Source: CAD feature listing. Evaluate the final solid. Frame: model axes, mm. Face numbers are marked on the shaded views. A direction names the side the tool comes from. Coordinates: 2 decimals unless noted, no trailing zeros. Loops run counter-clockwise (first coordinate to the right, second up) from the corner with the lowest first, then second, coordinate; pieces in that order, holes last. Notation, with made-up numbers: (56.5, 30.25) -> (92.5, 30.25) arc R19 ccw to (92.5, 41.25) -> close; hole circle Ø2 at (-39, 14.25). An arc over 180 degrees is marked (long way). Answer as a JSON object with one key per item and string values. Group by question number.
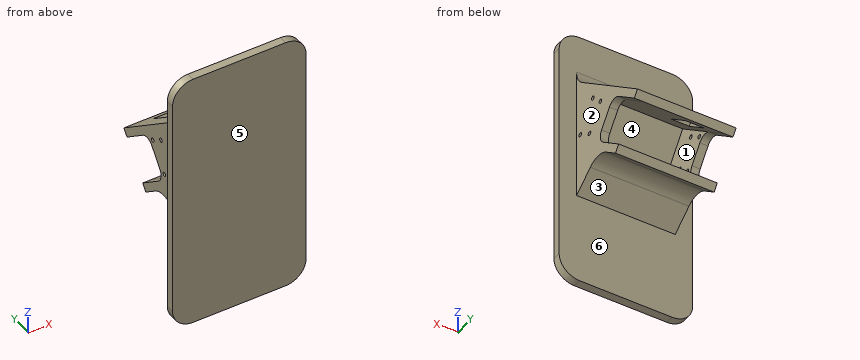
from build123d import *

# Parameters (mm, degrees)
BASE_PLATE_EXTRUDE_DEPTH    = 4
MOTORCASEEXTRUDE_DEPTH      = 24
MOTORCASEEXTRUDE_DEPTH_BACK = 24
SKETCH7_W                   = 40
SKETCH7_H                   = 20
CUT_EXTRUDE1_DEPTH          = 44
SKETCH9_W                   = 48
SKETCH9_H                   = 4
CUT_EXTRUDE2_DEPTH          = 28
FILLET_2_DEPTH              = 48
SKETCH11_W                  = 9
SKETCH11_H                  = 14
HOLE_FOR_WIRE_DEPTH         = 4
CUT_EXTRUDE3_REACH          = 14.5
SKETCH13_R                  = 1
CUT_EXTRUDE4_REACH          = 14.5
SKETCH14_R                  = 1


with BuildPart() as part:
    # Sketch1 → base_plate_extrude (new body)
    with BuildSketch(Plane(origin=(0, 0, 0), x_dir=(1, 0, 0), z_dir=(0, 1, 0))):
        with BuildLine():
            Line((-22.5, -63.5), (22.5, -63.5))
            ThreePointArc((22.5, -63.5), (29.571067812, -60.571067812), (32.5, -53.5))
            Line((32.5, -53.5), (32.5, 53.5))
            ThreePointArc((32.5, 53.5), (29.571067812, 60.571067812), (22.5, 63.5))
            Line((22.5, 63.5), (-22.5, 63.5))
            ThreePointArc((-22.5, 63.5), (-29.571067812, 60.571067812), (-32.5, 53.5))
            Line((-32.5, 53.5), (-32.5, -53.5))
            ThreePointArc((-32.5, -53.5), (-29.571067812, -60.571067812), (-22.5, -63.5))
        make_face()
    extrude(amount=BASE_PLATE_EXTRUDE_DEPTH)

    # Sketch5 → MotorCaseExtrude (add, two sides)
    with BuildSketch(Plane.ZY) as motorcaseextrude_sk:
        with BuildLine():
            Line((31.511856475, 15.127443917), (2.840895128, 53.623884992))
            Line((2.840895128, 53.623884992), (-19.615362165, 36.89915754))
            Line((-19.615362165, 36.89915754), (-11.812816694, 26.422695717))
            ThreePointArc((-11.812816694, 26.422695717), (-9.832908585, 20.44957877), (-11.812816694, 14.476461823))
            Line((-11.812816694, 14.476461823), (-19.615362165, 4))
            Line((-19.615362165, 4), (39.799233322, 4))
            Line((39.799233322, 4), (44.820226981, 4))
            ThreePointArc((44.820226981, 4), (40.333088108, 5.063245291), (36.80013509, 8.026883053))
            Line((36.80013509, 8.026883053), (31.511856475, 15.127443917))
        make_face()
    extrude(amount=MOTORCASEEXTRUDE_DEPTH)
    extrude(motorcaseextrude_sk.sketch, amount=-MOTORCASEEXTRUDE_DEPTH_BACK)

    # Sketch7 → Cut-Extrude1 (cut)
    with BuildSketch(Plane(origin=(0, 33.130958404, -24.674915427), x_dir=(1, 0, 0), z_dir=(0, 0.802009189, -0.597311695))):
        with Locations((0, -20.308597621)):
            Rectangle(SKETCH7_W, SKETCH7_H)
    extrude(amount=-CUT_EXTRUDE1_DEPTH, mode=Mode.SUBTRACT)

    # Sketch9 → Cut-Extrude2 (cut)
    with BuildSketch(Plane(origin=(0, 20.492926589, 27.515810556), x_dir=(1, 0, 0), z_dir=(0, 0.597311695, 0.802009189))):
        with Locations((0, 39.309948633)):
            Rectangle(SKETCH9_W, SKETCH9_H)
    extrude(amount=-CUT_EXTRUDE2_DEPTH, mode=Mode.SUBTRACT)

    # Sketch10 → fillet 2 (cut)
    with BuildSketch(Plane.ZY.offset(24)):
        with BuildLine():
            Line((-14.01807863, 36.080367563), (2.022105151, 48.026601457))
            Line((2.022105151, 48.026601457), (10.981780572, 35.996463621))
            ThreePointArc((10.981780572, 35.996463621), (11.919081057, 32.286190216), (9.9582931, 28.999859202))
            Line((9.9582931, 28.999859202), (1.93820121, 23.026742255))
            ThreePointArc((1.93820121, 23.026742255), (-1.772072196, 22.08944177), (-5.058403209, 24.050229727))
            Line((-5.058403209, 24.050229727), (-14.01807863, 36.080367563))
        make_face()
    extrude(amount=-FILLET_2_DEPTH, mode=Mode.SUBTRACT)

    # Sketch11 → Hole for wire (cut)
    with BuildSketch(Plane(origin=(0, 20.492926589, 27.515810556), x_dir=(1, 0, 0), z_dir=(0, 0.597311695, 0.802009189))):
        with Locations((-9.5, 22.309948633)):
            Rectangle(SKETCH11_W, SKETCH11_H)
    extrude(amount=-HOLE_FOR_WIRE_DEPTH, mode=Mode.SUBTRACT)

    # Sketch13 → Cut-Extrude3 (cut, up to next)
    with BuildSketch(Plane(origin=(-20, 0, 0), x_dir=(0, 0, -1), z_dir=(1, 0, 0)), mode=Mode.PRIVATE) as cut_extrude3_sk1:
        with Locations((-6.306750122, 13.811617607)):
            Circle(SKETCH13_R)
    cut_extrude3_tool1 = extrude(cut_extrude3_sk1.sketch, amount=-CUT_EXTRUDE3_REACH, mode=Mode.PRIVATE) & part.part
    add(cut_extrude3_tool1.solids().sort_by_distance((-20, 13.811618, 6.30675))[0], mode=Mode.SUBTRACT)
    # Sketch13 → Cut-Extrude3 (cut, up to next)
    with BuildSketch(Plane(origin=(-20, 0, 0), x_dir=(0, 0, -1), z_dir=(1, 0, 0)), mode=Mode.PRIVATE) as cut_extrude3_sk2:
        with Locations((-1.425907817, 19.528030678)):
            Circle(SKETCH13_R)
    cut_extrude3_tool2 = extrude(cut_extrude3_sk2.sketch, amount=-CUT_EXTRUDE3_REACH, mode=Mode.PRIVATE) & part.part
    add(cut_extrude3_tool2.solids().sort_by_distance((-20, 19.528031, 1.425908))[0], mode=Mode.SUBTRACT)
    # Sketch13 → Cut-Extrude3 (cut, up to next)
    with BuildSketch(Plane(origin=(-20, 0, 0), x_dir=(0, 0, -1), z_dir=(1, 0, 0)), mode=Mode.PRIVATE) as cut_extrude3_sk3:
        with Locations((-13.456045653, 28.487706099)):
            Circle(SKETCH13_R)
    cut_extrude3_tool3 = extrude(cut_extrude3_sk3.sketch, amount=-CUT_EXTRUDE3_REACH, mode=Mode.PRIVATE) & part.part
    add(cut_extrude3_tool3.solids().sort_by_distance((-20, 28.487706, 13.456046))[0], mode=Mode.SUBTRACT)
    # Sketch13 → Cut-Extrude3 (cut, up to next)
    with BuildSketch(Plane(origin=(-20, 0, 0), x_dir=(0, 0, -1), z_dir=(1, 0, 0)), mode=Mode.PRIVATE) as cut_extrude3_sk4:
        with Locations((-17.534878769, 22.173981333)):
            Circle(SKETCH13_R)
    cut_extrude3_tool4 = extrude(cut_extrude3_sk4.sketch, amount=-CUT_EXTRUDE3_REACH, mode=Mode.PRIVATE) & part.part
    add(cut_extrude3_tool4.solids().sort_by_distance((-20, 22.173981, 17.534879))[0], mode=Mode.SUBTRACT)

    # Sketch14 → Cut-Extrude4 (cut, up to next)
    with BuildSketch(Plane.ZY.offset(-20), mode=Mode.PRIVATE) as cut_extrude4_sk1:
        with Locations((10.283784148, 6.798641768)):
            Circle(SKETCH14_R)
    cut_extrude4_tool1 = extrude(cut_extrude4_sk1.sketch, amount=-CUT_EXTRUDE4_REACH, mode=Mode.PRIVATE) & part.part
    add(cut_extrude4_tool1.solids().sort_by_distance((20, 6.798642, 10.283784))[0], mode=Mode.SUBTRACT)
    # Sketch14 → Cut-Extrude4 (cut, up to next)
    with BuildSketch(Plane.ZY.offset(-20), mode=Mode.PRIVATE) as cut_extrude4_sk2:
        with Locations((23.115931173, 16.355628883)):
            Circle(SKETCH14_R)
    cut_extrude4_tool2 = extrude(cut_extrude4_sk2.sketch, amount=-CUT_EXTRUDE4_REACH, mode=Mode.PRIVATE) & part.part
    add(cut_extrude4_tool2.solids().sort_by_distance((20, 16.355629, 23.115931))[0], mode=Mode.SUBTRACT)
    # Sketch14 → Cut-Extrude4 (cut, up to next)
    with BuildSketch(Plane.ZY.offset(-20), mode=Mode.PRIVATE) as cut_extrude4_sk3:
        with Locations((6.307299779, 13.812026975)):
            Circle(SKETCH14_R)
    cut_extrude4_tool3 = extrude(cut_extrude4_sk3.sketch, amount=-CUT_EXTRUDE4_REACH, mode=Mode.PRIVATE) & part.part
    add(cut_extrude4_tool3.solids().sort_by_distance((20, 13.812027, 6.3073))[0], mode=Mode.SUBTRACT)
    # Sketch14 → Cut-Extrude4 (cut, up to next)
    with BuildSketch(Plane.ZY.offset(-20), mode=Mode.PRIVATE) as cut_extrude4_sk4:
        with Locations((17.535428426, 22.174390701)):
            Circle(SKETCH14_R)
    cut_extrude4_tool4 = extrude(cut_extrude4_sk4.sketch, amount=-CUT_EXTRUDE4_REACH, mode=Mode.PRIVATE) & part.part
    add(cut_extrude4_tool4.solids().sort_by_distance((20, 22.174391, 17.535428))[0], mode=Mode.SUBTRACT)


solid = part.part
1. Pin query (flat end, axial travel): pin 1 Ø15.5 at (y, z) = (22.5, 9.5) entering from -X; pin 2 Ø2.5 at (y, z) = (6.8, 10.28) entering from +X; pin 3 Ø1.8 at (y, z) = (19.53, 1.43) entering from -X. Return the tip coordinate at first contact, or that it passes through.
2. Section query D-D on y = 10. Return loops of the section in (x, z).
3. Section query A-A on x = -8. Return loops of the section in (y, z).
4. Ray query, L1, parallel to X at y = 13.5, z = 8.5; L2, parallel to Y at x = -29, z = 50; L3, parallel to Z at x = 8, y = 18.5. Return the intervals inside material, ascending.
5. Mould query, pull axis Y, two halves, no side actions, for the marked faces 4, 5 and 6. Classes: pulls with the +Y half, pulls with the -Y half, needs draft (parallel to the pull), parting line crosses it, or undercut.
6. Reachability of the marked faces 1, 2 and 3 from +Z, -Z, +X, -X, +Y, -Y: full face, straight path, thin tool, end or side. Return the list, or none.
7. Section query B-B on x = 16. Return loops of the section in (y, z), then the cut area to 3 significant figures.
8. Section query C-C on z = 43. Return loops of the section in (x, y), then the cut area to 3 significant figures.
Solved:
{
 "1": {"pin 1": "x = -24", "pin 2": "x = 24", "pin 3": "x = 20"},
 "2": {"outline": "(-24, -15.15) -> (24, -15.15) -> (24, 35.33) -> (-24, 35.33) -> close; hole (-20, 5.41) -> (20, 5.41) -> (20, 17.93) -> (-20, 17.93) -> close"},
 "3": {"outline": "(0, -63.5) -> (4, -63.5) -> (4, -19.62) -> (14.48, -11.81) arc R10 cw to (26.42, -11.81) -> (33.69, -17.23) -> (36.08, -14.02) -> (4, 9.87) -> (15.95, 25.91) -> (30.38, 15.16) -> (32.77, 18.37) -> (8.03, 36.8) arc R10 cw to (4, 44.82) -> (4, 63.5) -> (0, 63.5) -> close; (41.61, 6.8) -> (48.03, 2.02) -> (50.42, 5.23) -> (44, 10.01) -> close"},
 "4": {"L1": "-24 to -20, 20 to 24", "L2": "0 to 4", "L3": "-10.02 to -0.92, 24.01 to 29"},
 "5": {"face 4": "undercut", "face 5": "pulls with the -Y half", "face 6": "pulls with the +Y half"},
 "6": {"face 1": "none", "face 2": "+Z, -Z, +X, +Y", "face 3": "-Z, +X, -X"},
 "7": {"outline": "(0, -63.5) -> (4, -63.5) -> (4, -19.62) -> (14.48, -11.81) arc R10 cw to (26.42, -11.81) -> (33.69, -17.23) -> (36.08, -14.02) -> (4, 9.87) -> (15.95, 25.91) -> (48.03, 2.02) -> (50.42, 5.23) -> (8.03, 36.8) arc R10 cw to (4, 44.82) -> (4, 63.5) -> (0, 63.5) -> close", "area": "1,250 mm^2"},
 "8": {"outline": "(-32.5, 0) -> (32.5, 0) -> (32.5, 4) -> (24, 4) -> (24, 4.17) -> (-24, 4.17) -> (-24, 4) -> (-32.5, 4) -> close", "area": "268 mm^2"}
}
